The listing builds one solid part. Answer for the finished solid, in the listing's coordinates (mm). A direction names the side the tool comes from. Round coordinates to 2 decimals unless told otherwise and drop trailing zeros. Loops run counter-clockwise (first coordinate to the right, second up) from the corner with the lowest first, then second, coordinate; pieces in that order, holes last. Notation, with made-up numbers: (29, 58) - (85, 58) arc R14 ccw to (85, 68) - close; hole circle Ø3 at (23.25, -31). An arc over 180 degrees is marked (long way). One line per item, written item: value.
```python
from build123d import *

# Parameters (mm, degrees)
ESQUISSE1_W        = 17
ESQUISSE1_H        = 10
ESQUISSE1_R        = 3
BOSS_EXTRU_1_DEPTH = 5
ESQUISSE2_W        = 17
ESQUISSE2_H        = 6
BOSS_EXTRU_2_DEPTH = 2
CONG_1_R           = 1


with BuildPart() as part:
    # Esquisse1 → Boss.-Extru.1 (new body)
    with BuildSketch(Plane.XY):
        with Locations((8.5, 5)):
            Rectangle(ESQUISSE1_W, ESQUISSE1_H)
        with Locations((12, 5)):
            Circle(ESQUISSE1_R, mode=Mode.SUBTRACT)
    extrude(amount=BOSS_EXTRU_1_DEPTH)

    # Esquisse2 → Boss.-Extru.2 (add)
    with BuildSketch(Plane(origin=(0, 0, 0), x_dir=(-1, 0, 0), z_dir=(0, 0, -1))):
        with Locations((-8.5, -3)):
            Rectangle(ESQUISSE2_W, ESQUISSE2_H)
    extrude(amount=-BOSS_EXTRU_2_DEPTH)

    # Congé1
    cong_1_edges = [part.edges().sort_by_distance(p)[0] for p in [
        (8.5, 0, 2),
    ]]
    fillet(cong_1_edges, radius=CONG_1_R)


solid = part.part
```
1) Consider L1, parallel to Z at x = 2.5, y = -4; L2, parallel to Y at x = 12, z = 1.65; L3, parallel to X at y = 7.25, z = 3.2. Determine where each line is inside the solid, lowest interval first.
Final values:
L1: 0 to 2
L2: -6 to 2, 8 to 10
L3: 0 to 10.02, 13.98 to 17
2) A cutting plane is placed at A-A on y = 5. Give the vertices of the cut face in (x, z).
Final values:
outline: (0, 0) - (9, 0) - (9, 5) - (0, 5) - close; (15, 0) - (17, 0) - (17, 5) - (15, 5) - close
3) For a pull along Y with two mould halves and no side action, classify faces 3 (the flat face through (8, 10, 2)), 4 (the cylindrical face through (9.6, 3.2, 2.5)), 5 (the flat face through (9, -6, 1)) as released by +Y, released by -Y, zero draft, split by the parting line, or undercut.
Final values:
face 3: released by +Y
face 4: undercut
face 5: released by -Y
4) For faces 1 (the flat face through (9, -3, 2)), 2 (the flat face through (8, 5, 5)), determine the directions among +Z, -Z, +X, -X, +Y, -Y from which every point of the face is accessible in a straight line to the end or side of a thin tool.
Final values:
face 1: +Z, +X, -X, -Y
face 2: +Z, +X, -X, +Y, -Y
5) Each of these flat-tipped pins is pushed along its axis until it touches: pin 1 Ø2.5 at (x, y) = (10.5, -4) entering from +Z; pin 2 Ø3 at (x, z) = (6.5, 4) entering from -Y; pin 3 Ø1.6 at (x, z) = (11, 4.5) entering from -Y. Where does it stop, or does it pass through?
Final values:
pin 1: z = 2
pin 2: y = -0.13
pin 3: y = 0
6) A cutting plane is placed at C-C on z = 0.7. Give the vertices of the cut face in (x, y), and give its area (3 significant figures).
Final values:
outline: (0, -6) - (17, -6) - (17, 10) - (0, 10) - close; hole circle Ø6 at (12, 5)
area: 244 mm2
7) A cutting plane is placed at B-B on x = 12. Give the vertices of the cut face in (y, z), and give its area (3 significant figures).
Final values:
outline: (-6, 0) - (2, 0) - (2, 5) - (0, 5) - (0, 3) arc R1 cw to (-1, 2) - (-6, 2) - close; (8, 0) - (10, 0) - (10, 5) - (8, 5) - close
area: 32.2 mm2
8) A cutting plane is placed at D-D on x = 1.75. Give the vertices of the cut face in (y, z), and give its area (3 significant figures).
Final values:
outline: (-6, 0) - (10, 0) - (10, 5) - (0, 5) - (0, 3) arc R1 cw to (-1, 2) - (-6, 2) - close
area: 62.2 mm2
